Could you check a few things on this model? Use its own coordinates, in mm. Face numbers are marked on the shaded views. A direction names the side the tool comes from. Give positions to 0.01 mm unless a question says otherwise; leave off trailing zeros. Loops run counter-clockwise (first coordinate to the right, second up) from the corner with the lowest first, then second, coordinate; pieces in that order, holes last. Notation, with made-up numbers: M -27,-8 L -18,-8 A31 ccw -18,31 Z; hole C -19.5,40 d5. An arc over 180 degrees is marked long. Answer in a Markdown table with one row per item. Add a question column.
1. If we section it at C-C on z = 11.25: List the corners of the cut face in (x, y) for me.
2. I'm going to push flat-ended pins straight in: pin 1 Ø1.5 at (x, z) = (6.5, 5.5) entering from +Y; pin 2 Ø6.5 at (x, y) = (5, 1.5) entering from +Z; pin 3 Ø2 at (y, z) = (-8.5, 11.5) entering from -X; pin 4 Ø1.5 at (x, y) = (8.5, 4.5) entering from +Z. Where does each tip first touch, or does it pass through?
3. Which directions (+Z, -Z, +X, -X, +Y, -Y) give clear straight access to the entire face, cutting with the end or side of a thin tool? Please do the marked faces 4, 5, 6 and 7.
4. If we section it at A-A on x = 0: Count the separate pieces of the cut face and the enclosed holes in it, then the cut area to 3 significant figures.
5. If we section it at D-D on x = -6: List the corners of the cut face in (y, z) for me.
6. I need wall thicknesses on line 1 along Y through (x, z) = (0, 5); line 2 along Y through (x, z) = (0, 11.9); line 3 along X through (y, z) = (0.75, 11). Which ranges of each line are inside material? Lowest first, please. Write a range as from..to.
7. Thinking about a two-plate mould opening in X: for the marked faces 1, 2 and 3, which applies, released by +X, released by -X, zero draft, split by the parting line, or undercut?
```python
from build123d import *

# Parameters (mm, degrees)
SKETCH_R        = 11
SKETCH_R_2      = 1.7
PAD_DEPTH       = 13
SKETCH003_R     = 1.5
POCKET001_DEPTH = 6.5
PAD001_DEPTH    = 2
SKETCH006_R     = 3
POCKET003_DEPTH = 2.5
CHAMFER_SIZE    = 1.2
CHAMFER001_SIZE = 1.2
CHAMFER002_SIZE = 1.2
CHAMFER003_SIZE = 1.2
SKETCH007_R     = 2.2
POCKET_DEPTH    = 6


with BuildPart() as part:
    # Sketch → Pad (new body)
    with BuildSketch(Plane.XY):
        Circle(SKETCH_R)
        with Locations((0, 6)):
            Circle(SKETCH_R_2, mode=Mode.SUBTRACT)
        with Locations((-6, 0)):
            Circle(SKETCH_R_2, mode=Mode.SUBTRACT)
        with Locations((6, 0)):
            Circle(SKETCH_R_2, mode=Mode.SUBTRACT)
        with Locations((0, -6)):
            Circle(SKETCH_R_2, mode=Mode.SUBTRACT)
    extrude(amount=PAD_DEPTH)

    # Sketch003 → Pocket001 (cut)
    with BuildSketch(Plane.XY.offset(13)):
        Circle(SKETCH003_R)
    extrude(amount=-POCKET001_DEPTH, mode=Mode.SUBTRACT)

    # Sketch004 → Pad001 (new body)
    with BuildSketch(Plane.XY.offset(13)):
        with BuildLine():
            Line((-8.09798, 6.683766), (-2.930842, 1.516629))
            ThreePointArc((-1.516629, 2.930842), (-2.333452, 2.333452), (-2.930842, 1.516629))
            Line((-6.683766, 8.09798), (-1.516629, 2.930842))
            ThreePointArc((-6.683766, 8.09798), (-7.424621, 7.424621), (-8.09798, 6.683766))
        make_face()
        with BuildLine():
            Line((2.930842, -1.516629), (8.09798, -6.683766))
            ThreePointArc((6.683766, -8.09798), (7.424621, -7.424621), (8.09798, -6.683766))
            Line((1.516629, -2.930842), (6.683766, -8.09798))
            ThreePointArc((1.516629, -2.930842), (2.333452, -2.333452), (2.930842, -1.516629))
        make_face()
        with BuildLine():
            ThreePointArc((8.09798, 6.683766), (7.424621, 7.424621), (6.683766, 8.09798))
            Line((1.516629, 2.930842), (6.683766, 8.09798))
            ThreePointArc((2.930842, 1.516629), (2.333452, 2.333452), (1.516629, 2.930842))
            Line((8.09798, 6.683766), (2.930842, 1.516629))
        make_face()
        with BuildLine():
            ThreePointArc((-2.930842, -1.516629), (-2.333452, -2.333452), (-1.516629, -2.930842))
            Line((-1.516629, -2.930842), (-6.683766, -8.09798))
            ThreePointArc((-8.09798, -6.683766), (-7.424621, -7.424621), (-6.683766, -8.09798))
            Line((-8.09798, -6.683766), (-2.930842, -1.516629))
        make_face()
    extrude(amount=PAD001_DEPTH)

    # Sketch006 → Pocket003 (cut)
    with BuildSketch(Plane.XY.offset(13)):
        with Locations((0, 6)):
            Circle(SKETCH006_R)
        with Locations((-6, 0)):
            Circle(SKETCH006_R)
        with Locations((6, 0)):
            Circle(SKETCH006_R)
        with Locations((0, -6)):
            Circle(SKETCH006_R)
    extrude(amount=-POCKET003_DEPTH, mode=Mode.SUBTRACT)

    # Chamfer
    chamfer_edges = [part.edges().sort_by_distance(p)[0] for p in [
        (-1.7, 6, 10.5),
    ]]
    chamfer(chamfer_edges, length=CHAMFER_SIZE)

    # Chamfer001
    chamfer001_edges = [part.edges().sort_by_distance(p)[0] for p in [
        (-7.7, 0, 10.5),
    ]]
    chamfer(chamfer001_edges, length=CHAMFER001_SIZE)

    # Chamfer002
    chamfer002_edges = [part.edges().sort_by_distance(p)[0] for p in [
        (-1.7, -6, 10.5),
    ]]
    chamfer(chamfer002_edges, length=CHAMFER002_SIZE)

    # Chamfer003
    chamfer003_edges = [part.edges().sort_by_distance(p)[0] for p in [
        (4.3, 0, 10.5),
    ]]
    chamfer(chamfer003_edges, length=CHAMFER003_SIZE)

    # Sketch007 → Pocket (cut)
    with BuildSketch(Plane(origin=(0, 0, 0), x_dir=(1, 0, 0), z_dir=(0, 0, -1))):
        Circle(SKETCH007_R)
    extrude(amount=-POCKET_DEPTH, mode=Mode.SUBTRACT)


solid = part.part
```
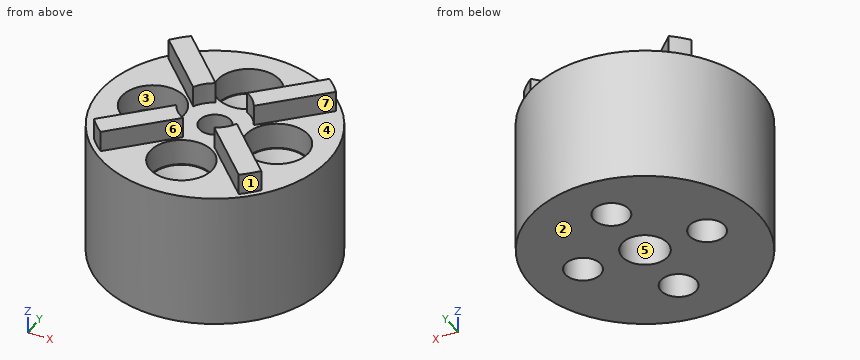
Results:
| question | item | result |
|---|---|---|
| 1 | outline | C 0,0 d22; hole C -6,0 d6; hole C 0,-6 d6; hole C 0,6 d6; hole C 0,0 d3; hole C 6,0 d6 |
| 2 | pin 1 | y = 9.38 |
| 2 | pin 2 | z = 15 |
| 2 | pin 3 | x = -8.05 |
| 2 | pin 4 | z = 13 |
| 3 | face 4 | +Z |
| 3 | face 5 | -Z |
| 3 | face 6 | +Z, -Y |
| 3 | face 7 | +Z, +X |
| 4 | separate pieces | 3 |
| 4 | enclosed holes | 0 |
| 4 | area | 136 mm2 |
| 5 | outline | M -9.22,0 L -1.7,0 L -1.7,9.3 L -2.9,10.5 L -3,10.5 L -3,13 L -4.59,13 L -4.59,15 L -7.41,15 L -7.41,13 L -9.22,13 Z; M 1.7,0 L 9.22,0 L 9.22,13 L 7.41,13 L 7.41,15 L 4.59,15 L 4.59,13 L 3,13 L 3,10.5 L 2.9,10.5 L 1.7,9.3 Z |
| 6 | line 1 | -11..-7.7, -4.3..-2.2, 2.2..4.3, 7.7..11 |
| 6 | line 2 | -11..-9, -3..-1.5, 1.5..3, 9..11 |
| 6 | line 3 | -10.97..-8.9, -3.1..-1.3, 1.3..3.1, 8.9..10.97 |
| 7 | face 1 | released by +X |
| 7 | face 2 | zero draft |
| 7 | face 3 | undercut |
